The model under review builds one solid part; all positions refer to its coordinate system, in mm. A direction names the side the tool comes from. Coordinates: 2 decimals unless noted, no trailing zeros. Loops run counter-clockwise (first coordinate to the right, second up) from the corner with the lowest first, then second, coordinate; pieces in that order, holes last. Notation, with made-up numbers: (88.5, 81) -> (130.5, 81) arc R37 ccw to (130.5, 117) -> close; hole circle Ø6 at (17, 37.5). An arc over 180 degrees is marked (long way). One line per question, with ' | ' between items. Start each with the question number.
Autodesk Inventor part; units mm, degrees
ref_plane "YZ Plane" through (0, 0, 0) normal (1, 0, 0) x (0, 1, 0)
ref_plane "XZ Plane" through (0, 0, 0) normal (0, 1, 0) x (-1, 0, 0)
ref_plane "XY Plane" through (0, 0, 0) normal (0, 0, 1) x (1, 0, 0)
sketch "Sketch1" plane through (0, 0, 0) normal (1, 0, 0) x (0, 1, 0)
  circle A0 centre (0, 0) radius 8
  line L0 (0, 20) -> (0, 0) construction
  arc A1 (5.9699, 20.6) -> (-5.9699, 20.6) centre (0, 20) ccw
  line L1 (-7.9599, 0.8) -> (-5.9699, 20.6)
  line L2 (7.9599, 0.8) -> (5.9699, 20.6)
  line L3 (-5.3312, 5.9647) -> (7.8312, -1.6346) construction
  line L4 (5.3312, -5.9647) -> (-7.8312, 1.6346) construction
  line L5 (-6.9282, 4) -> (6.9282, -4) construction
  line L6 (-5.3116, 5.9823) -> (7.8366, -1.6088)
  line L7 (-7.8366, 1.6088) -> (5.3116, -5.9823)
  line L8 (5.3312, 5.9647) -> (-7.8312, -1.6346) construction
  line L9 (-5.3312, -5.9647) -> (7.8312, 1.6346) construction
  line L10 (6.9282, 4) -> (-6.9282, -4) construction
  line L11 (5.3116, 5.9823) -> (-7.8366, -1.6088)
  line L12 (7.8366, 1.6088) -> (-5.3116, -5.9823)
  line L13 (-7.5911, 2.525) -> (7.5911, 2.525)
  line L14 (-7.5993, 2.5) -> (7.5993, 2.5) construction
  line L15 (-8, 0) -> (8, 0) construction
  line L16 (-7.5911, -2.525) -> (7.5911, -2.525)
  line L17 (-7.5993, -2.5) -> (7.5993, -2.5) construction
  point P0 (7.9599, 0.8)
  point P1 (-5.3116, -5.9823)
  point P2 (0, -2.9156)
  point P3 (5.3116, -5.9823)
  point P4 (5.05, 0)
  point P5 (7.8366, 1.6088)
  point P6 (5.3116, 5.9823)
  point P7 (0, 2.9156)
  point P8 (-7.8366, 1.6088)
  point P9 (-5.05, 0)
  point P10 (-7.8366, -1.6088)
  dimension "d0" = 16
  dimension "d1" = 20
  dimension "d2" = 12
  dimension "d28" = 60
  dimension "d29" = 5
  dimension "d30" = 0.025
  dimension "d31" = 5
  dimension "d32" = 0.025
extrude "Extrusion1" add sketch "Sketch1" against normal blind 6
extrude "Extrusion2" cut sketch "Sketch1" against normal blind 3 contours A0 L1 A1 L2
hole "M4" at (0, 0, 20) direction (-1, 0, 0) diameter 3.242 end through all
hole "Phi3.2" at (0, 0, 0) direction (-1, 0, 0) diameter 3.2 end through all
equation "\"d31\" = d29"
equation "\"d32\" = d30"
properties part number "LongCrankFrameBasis" material "Aluminum 7075"
1) Insertion check: pin 1 Ø3 at (x, z) = (-4.5, 11) entering from +Y; pin 2 Ø2 at (x, y) = (-3, 1.5) entering from -Z; pin 3 Ø1 at (x, z) = (-4.5, -1.5) entering from +Y; pin 4 Ø5 at (y, z) = (0, 0) entering from +X. Each pin has a flat end and moves straight along its axis. Give the tip position at first contact, or say it passes through.
2) Machinability: for faces 1 (the face through (-4.48, 6.98, 10.56)), 2 (the face through (-2.291, -0.945, -7.944)), which of the approach directions +Z, -Z, +X, -X, +Y, -Y give a long, thin tool a straight path to every point of the face, cutting with its end or side? Answer none if there is none.
3) Consider section B-B, the plane x = -3.75. Write out the cut boundary in (y, z), plus the area to 3 significant figures.
4) Consider section D-D, the plane z = 3.5. Write out the cut boundary in (x, y).
5) Consider section C-C, the plane y = 0. Write out the cut boundary in (x, z), plus the area to 3 significant figures.
6) Wall thickness on L1, parallel to Y at x = -3.45, z = 0; L2, parallel to X at y = -1, z = 10.5: over which ranges is each line inside the solid? List them lowest first.
7) Consider section A-A, the plane z = 0. Write out the cut boundary in (x, y).
Filled sheet:
1) pin 1: y = 7.09 | pin 2: z = -7.98 | pin 3: y = 7.94 | pin 4: x = 0
2) face 1: +Z, +X, -X, +Y | face 2: +X
3) outline: (-7.96, 0.8) arc R8 ccw (long way) to (7.96, 0.8) -> (5.97, 20.6) arc R6 ccw to (-5.97, 20.6) -> close; hole circle Ø3.24 at (0, 20); hole circle Ø3.2 at (0, 0) | area: 422 mm^2
4) outline: (-6, -7.69) -> (-3, -7.69) -> (-3, -7.19) -> (0, -7.19) -> (0, 7.19) -> (-3, 7.19) -> (-3, 7.69) -> (-6, 7.69) -> close
5) outline: (-6, -8) -> (0, -8) -> (0, -1.6) -> (-6, -1.6) -> close; (-6, 1.6) -> (0, 1.6) -> (0, 8) -> (-3, 8) -> (-3, 18.38) -> (-6, 18.38) -> close; (-6, 21.62) -> (-3, 21.62) -> (-3, 26) -> (-6, 26) -> close | area: 121 mm^2
6) L1: -8 to -1.6, 1.6 to 8 | L2: -6 to -3
7) outline: (-6, -8) -> (0, -8) -> (0, -1.6) -> (-6, -1.6) -> close; (-6, 1.6) -> (0, 1.6) -> (0, 8) -> (-6, 8) -> close
